Autodesk Inventor part; units mm, degrees
ref_plane "YZ Plane" through (0, 0, 0) normal (1, 0, 0) x (0, 1, 0)
ref_plane "XZ Plane" through (0, 0, 0) normal (0, 1, 0) x (-1, 0, 0)
ref_plane "XY Plane" through (0, 0, 0) normal (0, 0, 1) x (1, 0, 0)
sketch "Sketch1" plane through (0, 0, 0) normal (1, 0, 0) x (0, 1, 0)
  line L0 (0, 0) -> (41.275, 0)
  line L1 (41.275, 0) -> (41.275, -19.05)
  line L2 (41.275, -19.05) -> (0, -19.05)
  line L3 (0, -19.05) -> (0, 0)
  dimension "d0" = 41.275
  dimension "d1" = 19.05
extrude "Extrusion1" add sketch "Sketch1" along normal blind 3.175
sketch "Sketch2" plane through (3.175, 0, 0) normal (1, 0, 0) x (0, 0, -1)
  line L0 (0, 41.275) -> (0, 0)
  line L1 (0, 0) -> (19.05, 0)
  line L2 (19.05, 0) -> (19.05, 41.275)
  line L3 (19.05, 41.275) -> (0, 41.275)
  line L4 (5.2917, 41.275) -> (13.7583, 41.275)
  line L5 (13.7583, 41.275) -> (13.7583, 44.45)
  line L6 (13.7583, 44.45) -> (5.2917, 44.45)
  line L7 (5.2917, 44.45) -> (5.2917, 41.275)
  line L8 (19.05, 29.6333) -> (22.225, 29.6333)
  line L9 (22.225, 29.6333) -> (22.225, 14.8167)
  line L10 (22.225, 14.8167) -> (19.05, 14.8167)
  line L11 (19.05, 14.8167) -> (19.05, 29.6333)
  line L12 (0, 29.6333) -> (-3.175, 29.6333)
  line L13 (-3.175, 29.6333) -> (-3.175, 14.8167)
  line L14 (-3.175, 14.8167) -> (0, 14.8167)
  line L15 (0, 14.8167) -> (0, 29.6333)
  dimension "d4" = 8.4667
  dimension "d5" = 3.175
  dimension "d6" = 5.2917
  dimension "d7" = 3.175
  dimension "d8" = 14.8167
  dimension "d9" = 3.175
  dimension "d10" = 14.8167
  dimension "d11" = 14.8167
extrude "Extrusion2" add sketch "Sketch2" against normal blind 3.175 contours L0 L14 L13 L12 | L7 L6 L5 L3 | L8 L9 L10 L2
sketch "Sketch3" plane through (3.175, 0, 0) normal (1, 0, 0) x (0, 0, -1)
  line L0 (-3.175, 29.6333) -> (-3.175, 14.8167)
  line L1 (0, 0) -> (19.05, 0)
  circle A0 centre (9.525, 8.89) radius 3.5052
  circle A1 centre (16.1036, 8.89) radius 0.889
  circle A2 centre (2.9464, 8.89) radius 0.889
  dimension "d14" = 7.0104
  dimension "d15" = 12.7
  dimension "d16" = 8.89
  dimension "d17" = 1.778
  dimension "d18" = 1.778
  dimension "d19" = 13.1572
  dimension "d20" = 6.5786
extrude "Extrusion3" cut sketch "Sketch3" against normal blind 3.175
equation "\"d0\" = angleHeight - thick"
equation "\"d1\" = angleDepth - 2 * thick"
equation "\"d2\" = thick"
equation "\"d4\" = 0.333333 * angleDepth"
equation "\"d5\" = thick"
equation "\"d6\" = 0.333333 * angleDepth - thick"
equation "\"d7\" = thick"
equation "\"d8\" = 0.333333 * angleHeight"
equation "\"d9\" = thick"
equation "\"d10\" = 0.333333 * angleHeight"
equation "\"d11\" = 0.333333 * angleHeight"
equation "\"d12\" = thick"
equation "\"d14\" = hornCenter"
equation "\"d15\" = 0.5 * angleDepth"
equation "\"d16\" = hornOffset"
equation "\"d17\" = hornHole"
equation "\"d18\" = hornHole"
equation "\"d19\" = hornDia"
equation "\"d20\" = 0.5 * hornDia"
equation "\"d21\" = thick"
equation "\"angleHeight\" = 44.45"
equation "\"angleDepth\" = 25.4"
equation "\"hornCenter\" = 7.0104"
equation "\"hornOffset\" = 8.89"
equation "\"thick\" = 3.175"
equation "\"hornHole\" = 1.778"
equation "\"hornDia\" = 13.1572"
properties part number "AngleLower"
Work out the finished part from the listing and answer in its coordinate system (mm). A direction names the side the tool comes from. Give positions to 0.01 mm unless a question says otherwise; leave off trailing zeros. Write each loop counter-clockwise with the first axis right and the second up, starting at its lowest first coordinate (ties: lowest second). Pieces come first, ordered by that corner, then holes.
(1) The part is cut by section D-D on z = -20.5. Write down the section's boundary in (x, y) (3 decimals), plus the area to 3 significant figures.
Final values:
outline: (0, 14.817) - (3.175, 14.817) - (3.175, 29.633) - (0, 29.633) - close
area: 47.0 mm2
(2) Which of the six approach directions +Z, -Z, +X, -X, +Y, -Y give full straight-line access (tool end or side, diameter ignored) to faces 1 (the flat face through (2, 41.275, -16)), 2 (the flat face through (2, 8, -19.05)), 3 (the flat face through (2, 14.817, 2)), 4 (the flat face through (2, 43, -5.292)), 5 (the flat face through (3.175, 22, -9))?
Final values:
face 1: -Z, +X, -X, +Y
face 2: -Z, +X, -X, -Y
face 3: +Z, +X, -X, -Y
face 4: +Z, +X, -X, +Y
face 5: +Z, -Z, +X, +Y, -Y
(3) The part is cut by section B-B on z = -16. Write down the section's boundary in (x, y) (3 decimals).
Final values:
outline: (0, 0) - (3.175, 0) - (3.175, 8.007) - (0, 8.007) - close; (0, 9.773) - (3.175, 9.773) - (3.175, 41.275) - (0, 41.275) - close
(4) The part is cut by section C-C on x = 1. Write down the section's boundary in (y, z) (3 decimals).
Final values:
outline: (0, -19.05) - (14.817, -19.05) - (14.817, -22.225) - (29.633, -22.225) - (29.633, -19.05) - (41.275, -19.05) - (41.275, -13.758) - (44.45, -13.758) - (44.45, -5.292) - (41.275, -5.292) - (41.275, 0) - (29.633, 0) - (29.633, 3.175) - (14.817, 3.175) - (14.817, 0) - (0, 0) - close; hole circle Ø7.01 at (8.89, -9.525); hole circle Ø1.778 at (8.89, -16.104); hole circle Ø1.778 at (8.89, -2.946)
(5) Flat-ended cylindrical pins translate along their axes: pin 1 Ø1 at (x, z) = (1.5, -3.5) entering from +Y (3 decimals); pin 2 Ø1 at (x, y) = (1.5, 33) entering from -Z; pin 3 Ø1 at (x, y) = (2, 42.5) entering from -Z. Find the tip coordinate at first contact, or state that the pin passes through.
Final values:
pin 1: stops at y = 41.275
pin 2: stops at z = -19.05
pin 3: stops at z = -13.76
(6) The mould has two halves that part along Z. Classify faces 6 (the cylindrical face through (1.61, 5.78, -11.14)), 7 (the flat face through (2, 29.633, 2)), 8 (the flat face through (2, 35, 0)): pulls with the +Z half, pulls with the -Z half, needs draft (parallel to the pull), parting line crosses it, or undercut.
Final values:
face 6: undercut
face 7: needs draft
face 8: pulls with the +Z half
(7) Straight lines are drawn through the part: line 1 (Z direction, x = 0.35, y = 9); line 2 (Y direction, x = 1.95, z = -3) (3 decimals); line 3 (Z direction, x = 1.35, y = 4). For each, find the intervals that lie inside material, in ascending order.
Final values:
line 1: z = -19.05 to -16.99, -15.22 to -13.03, -6.02 to -3.83, -2.06 to 0
line 2: y = 0 to 8.003, 9.777 to 41.275
line 3: z = -19.05 to 0
(8) The part is cut by section A-A on y = 8.89. Write down the section's boundary in (x, z) (3 decimals), plus the area to 3 significant figures.
Final values:
outline: (0, -19.05) - (3.175, -19.05) - (3.175, -16.993) - (0, -16.993) - close; (0, -15.215) - (3.175, -15.215) - (3.175, -13.03) - (0, -13.03) - close; (0, -6.02) - (3.175, -6.02) - (3.175, -3.835) - (0, -3.835) - close; (0, -2.057) - (3.175, -2.057) - (3.175, 0) - (0, 0) - close
area: 26.9 mm2
